Read the model definition and answer for the solid it produces. Units are mm, in the model's axes. A direction names the side the tool comes from. Give positions to 0.01 mm unless a question says otherwise; leave off trailing zeros. Order: outer loops, then holes, each group sorted by start corner. A loop starts at its lowest first (then second) coordinate and runs counter-clockwise, first axis right, second up. Notation, with made-up numbers: (71.5, 11) - (91.5, 11) arc R26 cw to (91.5, 29) - close; hole circle Ø2 at (72.5, 1.5). An arc over 180 degrees is marked (long way). Use a Markdown table: item, result. Add a question column.
1. Consider L1, parallel to Y at x = 2, z = -4.5; L2, parallel to Y at x = -1, z = -18; L3, parallel to X at y = 77, z = 11.5. Determine where each line is inside the solid, lowest interval first.
2. A cutting plane is placed at C-C on z = 34.5. Determine the outline of the cut face in (x, y).
3. Which of the six approach directions +Z, -Z, +X, -X, +Y, -Y give full straight-line access (tool end or side, diameter ignored) to faces 4 (the flat face through (-4, 20, 1)), 5 (the flat face through (-20, 10, 20))?
4. A cutting plane is placed at B-B on z = 13. Determine the outline of the cut face in (x, y).
5. A cutting plane is placed at D-D on y = 81. Determine the outline of the cut face in (x, z).
6. A cutting plane is placed at A-A on x = -13. Determine the outline of the cut face in (y, z), and give its area (3 significant figures).
7. Flat-ended cylindrical pins translate along their axes: P1, Ø10, axis at y = 34, z = -3.5, coming from the -X side; P2, Ø12, axis at y = 54, z = 1.5, coming from the -X side; P3, Ø1.5, axis at y = 73.5, z = 7, coming from the -X side. Find the tip coordinate at first contact, or state that the pin passes through.
8. For a pull along Y with two mould halves and no side action, classify faces 1 (the flat face through (-20, 10, -20)), 2 (the flat face through (1, 90, 1)), 3 (the flat face through (20, 30, 0)) as released by +Y, released by -Y, zero draft, split by the parting line, or undercut.
Autodesk Inventor part; units mm, degrees
ref_plane "YZ Plane" through (0, 0, 0) normal (1, 0, 0) x (0, 1, 0)
ref_plane "XZ Plane" through (0, 0, 0) normal (0, 1, 0) x (-1, 0, 0)
ref_plane "XY Plane" through (0, 0, 0) normal (0, 0, 1) x (1, 0, 0)
sketch "Эскиз1" plane through (0, 0, 0) normal (0, 1, 0) x (-1, 0, 0)
  circle A0 centre (0, 0) radius 40
  line L0 (0, 40) -> (40, 0)
  line L1 (40, 0) -> (0, -40)
  line L2 (0, -40) -> (-40, 0)
  line L3 (-40, 0) -> (0, 40)
  dimension "d0" = 80
extrude "Выдавливание1" add sketch "Эскиз1" along normal blind 90 contours L1 L2 L3 L0
sketch "Эскиз2" plane through (0, 0, 0) normal (0, 0, 1) x (1, 0, 0)
  line L0 (0, 90) -> (-40, 90)
  line L1 (-40, 90) -> (-40, 70)
  line L2 (-40, 0) -> (-40, 90)
  line L3 (0, 0) -> (-40, 0)
  line L4 (-40, 0) -> (-40, 20)
  line L5 (-40, 20) -> (20, 20)
  line L6 (20, 20) -> (20, 40)
  line L7 (20, 40) -> (-40, 70)
  line L8 (-40, 20) -> (-40, 70)
  dimension "d3" = 20
  dimension "d4" = 20
  dimension "d5" = 60
  dimension "d6" = 20
extrude "Выдавливание2" cut sketch "Эскиз2" against normal mid plane 90
properties part number "Деталь1Индивидуал"
Output values:
| question | item | result |
|---|---|---|
| 1 | L1 | 0 to 20, 49 to 90 |
| 1 | L2 | 0 to 20, 50.5 to 90 |
| 1 | L3 | -28.5 to 28.5 |
| 2 | outline | (-5.5, 0) - (5.5, 0) - (5.5, 20) - (-5.5, 20) - close; (-5.5, 52.75) - (5.5, 47.25) - (5.5, 90) - (-5.5, 90) - close |
| 3 | face 4 | +Z, -Z, -X |
| 3 | face 5 | +Z, -X, +Y, -Y |
| 4 | outline | (-27, 0) - (27, 0) - (27, 90) - (-27, 90) - (-27, 63.5) - (20, 40) - (20, 20) - (-27, 20) - close |
| 5 | outline | (-40, 0) - (0, -40) - (40, 0) - (0, 40) - close |
| 6 | outline | (0, -27) - (20, -27) - (20, 27) - (0, 27) - close; (56.5, -27) - (90, -27) - (90, 27) - (56.5, 27) - close |
| 6 | area | 2,890 mm² |
| 7 | P1 | x = 20 |
| 7 | P2 | x = -20 |
| 7 | P3 | x = -33.75 |
| 8 | face 1 | zero draft |
| 8 | face 2 | released by +Y |
| 8 | face 3 | undercut |
